Study the drawing (mm; zero at the part's minimum x, y, z) and answer. A direction names the side the tool comes from. Coordinates: 2 decimals unless noted, no trailing zeros. Order: outer loops, then holes, each group sorted by start corner. A loop starts at its lowest first (then second) coordinate and runs counter-clockwise, first axis right, second up.
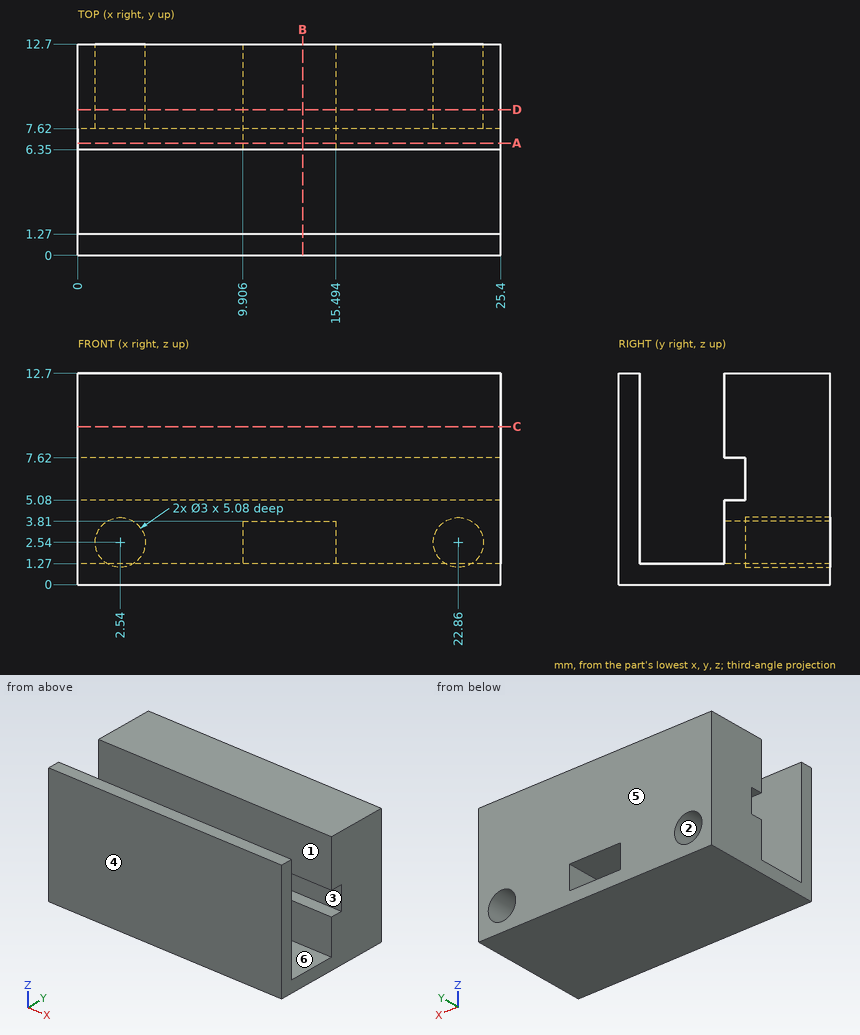
(1) Find section A-A on y = 6.75. Determine the outline of the cut face in (x, z), then the cut area to 3 significant figures.
(2) Find the intervals of material crossed by probe 1 along X at (y, z) = (8.8, 2.54); probe 2 along Y at (x, z) = (7, 3); probe 3 along X at (y, z) = (9, 1.5), in increasing order.
(3) Find section C-C on z = 9.5. Determine the outline of the cut face in (x, y).
(4) A tool of negligible diameter and unlimited length cuts with its end or side. For the marked faces 1, 2 and 3, from which of +Z, -Z, +X, -X, +Y, -Y can it reach the whole face along a straight path? Write none if from no direction.
(5) The mould has two halves that part along Y. Classify the marked faces 4, 5 and 6: pulls with the +Y half, pulls with the -Y half, needs draft (parallel to the pull), parting line crosses it, or undercut.
(6) Given pin 1 Ø3 at (x, z) = (18, 3) entering from -Y; pin 2 Ø1.5 at (x, z) = (3, 2) entering from +Y; pin 3 Ø1 at (y, z) = (5, 4) entering from -X, each flat-ended and moving along its own axis, determine where each tip first touches the part or whether it passes through.
(7) Find section B-B on x = 13.5. Determine the outline of the cut face in (y, z).
(8) Find section D-D on y = 8.75. Determine the outline of the cut face in (x, z).
Resolved:
1. outline: (0, 0) - (25.4, 0) - (25.4, 5.08) - (0, 5.08) - close; (0, 7.62) - (25.4, 7.62) - (25.4, 12.7) - (0, 12.7) - close; hole (9.91, 1.27) - (15.49, 1.27) - (15.49, 3.81) - (9.91, 3.81) - close
1. area: 244 mm2
2. probe 1: x = 0 to 1.04, 4.04 to 9.91, 15.49 to 21.36, 24.36 to 25.4
2. probe 2: y = 0 to 1.27, 6.35 to 12.7
2. probe 3: x = 0 to 1.46, 3.62 to 9.91, 15.49 to 21.78, 23.94 to 25.4
3. outline: (0, 0) - (25.4, 0) - (25.4, 1.27) - (0, 1.27) - close; (0, 6.35) - (25.4, 6.35) - (25.4, 12.7) - (0, 12.7) - close
4. face 1: +Z, +X, -X
4. face 2: +Y
4. face 3: +X, -X
5. face 4: pulls with the -Y half
5. face 5: pulls with the +Y half
5. face 6: undercut
6. pin 1: stops at y = 0
6. pin 2: stops at y = 7.62
6. pin 3: passes through
7. outline: (0, 0) - (12.7, 0) - (12.7, 1.27) - (1.27, 1.27) - (1.27, 12.7) - (0, 12.7) - close; (6.35, 3.81) - (12.7, 3.81) - (12.7, 12.7) - (6.35, 12.7) - (6.35, 7.62) - (7.62, 7.62) - (7.62, 5.08) - (6.35, 5.08) - close
8. outline: (0, 0) - (25.4, 0) - (25.4, 12.7) - (0, 12.7) - close; hole circle Ø3 at (2.54, 2.54); hole (9.91, 1.27) - (15.49, 1.27) - (15.49, 3.81) - (9.91, 3.81) - close; hole circle Ø3 at (22.86, 2.54)
